```python
from build123d import *

# Parameters (mm, degrees)
ESBO_O1_R                = 7.5
RESSALTO_EXTRUS_O1_DEPTH = 3
ESBO_O2_R                = 6
ESBO_O2_R_2              = 4.5
RESSALTO_EXTRUS_O2_DEPTH = 30


with BuildPart() as part:
    # Esboço1 → Ressalto-extrusão1 (new body)
    with BuildSketch(Plane.XY):
        Circle(ESBO_O1_R)
    extrude(amount=RESSALTO_EXTRUS_O1_DEPTH)

    # Esboço2 → Ressalto-extrusão2 (add)
    with BuildSketch(Plane.XY.offset(3)):
        Circle(ESBO_O2_R)
        Circle(ESBO_O2_R_2, mode=Mode.SUBTRACT)
    extrude(amount=RESSALTO_EXTRUS_O2_DEPTH)


solid = part.part
```
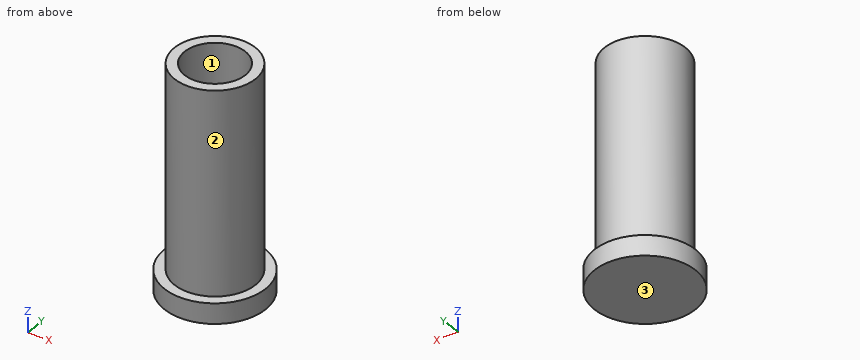
Work out the finished part from the listing and answer in its coordinate system (mm). Face numbers are marked on the shaded views. Give positions to 0.01 mm unless a question says otherwise; leave off trailing zeros. Order: outer loops, then holes, each group sorted by start corner. A loop starts at its lowest first (then second) coordinate and runs counter-clockwise, first axis right, second up. Notation, with made-up numbers: (80.5, 28.25) - (97.5, 28.25) arc R11 cw to (97.5, 42.25) - close; hole circle Ø4 at (-7, 13). An arc over 180 degrees is marked (long way). One line per item, written item: value. Start each with the question number.
1. Section D-D, the plane x = 5.5 is taken. Write down the section's boundary in (y, z), then the cut area to 3 significant figures.
2. Section C-C, the plane z = 29 is taken. Write down the section's boundary in (x, y).
3. Each of these flat-tipped pins is pushed along its axis until it touches: pin 1 Ø6 at (y, z) = (5.5, 4.5) entering from -X; pin 2 Ø4 at (y, z) = (-4, 19.5) entering from +X; pin 3 Ø2 at (y, z) = (5, 9) entering from +X; pin 4 Ø8 at (x, y) = (-2.5, -2.5) entering from -Z. Where does it stop, or does it pass through?
4. Section A-A, the plane x = 0 is taken. Write down the section's boundary in (y, z).
5. For a pull along Y with two mould halves and no side action, classify the marked faces 1, 2 and 3 as released by +Y, released by -Y, zero draft, split by the parting line, or undercut.
6. Consider line 1 (Y direction, x = 0, z = 21.5); line 2 (Y direction, x = -2.5, z = 5.5). Determine where each line is inside the solid, lowest interval first.
Filled sheet:
1. outline: (-5.1, 0) - (5.1, 0) - (5.1, 3) - (2.4, 3) - (2.4, 33) - (-2.4, 33) - (-2.4, 3) - (-5.1, 3) - close
1. area: 174 mm²
2. outline: circle Ø12 at (0, 0); hole circle Ø9 at (0, 0)
3. pin 1: x = -6.92
3. pin 2: x = 5.66
3. pin 3: x = 4.47
3. pin 4: z = 0
4. outline: (-7.5, 0) - (7.5, 0) - (7.5, 3) - (6, 3) - (6, 33) - (4.5, 33) - (4.5, 3) - (-4.5, 3) - (-4.5, 33) - (-6, 33) - (-6, 3) - (-7.5, 3) - close
5. face 1: undercut
5. face 2: split by the parting line
5. face 3: zero draft
6. line 1: -6 to -4.5, 4.5 to 6
6. line 2: -5.45 to -3.74, 3.74 to 5.45
